Geometry: final body of the model. Coordinates: model frame, mm. Give positions to 0.01 mm unless a question says otherwise; leave off trailing zeros. Loops run counter-clockwise (first coordinate to the right, second up) from the corner with the lowest first, then second, coordinate; pieces in that order, holes last. Notation, with made-up numbers: M 37,1.25 L 74,1.25 A30 ccw 74,30.25 Z; hole C -21.75,56 d2. An arc over 180 degrees is marked long. Put each result on its own line as item: value.
```python
from build123d import *

# Parameters (mm, degrees)
DELKA_DEPTH       = 250
D_RA1_D           = 3.5
D_RA1_CBORE_D     = 6
D_RA1_CBORE_DEPTH = 4.5
LINPOLE1_COUNT    = 10
LINPOLE1_PITCH    = 25


with BuildPart() as part:
    # Skica1 → Delka (new body)
    with BuildSketch(Plane(origin=(0, 0, 0), x_dir=(1, 0, 0), z_dir=(0, 1, 0))):
        with BuildLine():
            Line((-5.5, -8), (5.5, -8))
            Line((5.5, -8), (6, -7.5))
            Line((6, -7.5), (6, -6.661895004))
            ThreePointArc((6, -6.661895004), (5.52983318, -6.420240767), (5.209128789, -6))
            Line((5.209128789, -6), (4, -5.95))
            Line((4, -5.95), (4, -5.05))
            Line((4, -5.05), (5.209128789, -5))
            ThreePointArc((5.209128789, -5), (5.52983318, -4.579759233), (6, -4.338104996))
            Line((6, -4.338104996), (6, -0.5))
            Line((6, -0.5), (5.5, 0))
            Line((5.5, 0), (-1.6, 0))
            ThreePointArc((-1.6, 0), (-2, -0.2), (-2.4, 0))
            Line((-2.4, 0), (-5.5, 0))
            Line((-5.5, 0), (-6, -0.5))
            Line((-6, -0.5), (-6, -4.338104996))
            ThreePointArc((-6, -4.338104996), (-5.52983318, -4.579759233), (-5.209128789, -5))
            Line((-5.209128789, -5), (-4, -5.05))
            Line((-4, -5.05), (-4, -5.95))
            Line((-4, -5.95), (-5.209128789, -6))
            ThreePointArc((-5.209128789, -6), (-5.52983318, -6.420240767), (-6, -6.661895004))
            Line((-6, -6.661895004), (-6, -7.5))
            Line((-6, -7.5), (-5.5, -8))
        make_face()
    extrude(amount=DELKA_DEPTH)

    # Díra1 (through all)
    with Locations(Plane.XY.offset(8)):
        with Locations((0, 12.5)):
            d_ra1 = CounterBoreHole(D_RA1_D / 2, D_RA1_CBORE_D / 2, D_RA1_CBORE_DEPTH)

    # Zkosení1: read off the stored shape, not the designer's step
    # Zkosení1 outline → Zkosení1 (revolve, cut)
    with BuildSketch(Plane.XZ.offset(-12.5)):
        Polygon((2.050001495, -1.495e-06), (1.75, 0.3), (1.75, -1.495e-06), align=None)
        Polygon((3, 8), (3, 7.7), (3.3, 8), align=None)
    zkosen_1 = revolve(axis=Axis((0, 12.5, 0), (0, 0, 1)), mode=Mode.SUBTRACT)

    # LinPole1: Díra1, Zkosení1 ×10
    with Locations(*[(0, i * LINPOLE1_PITCH, 0) for i in range(1, LINPOLE1_COUNT)]):
        add(d_ra1, mode=Mode.SUBTRACT)
        add(zkosen_1, mode=Mode.SUBTRACT)


solid = part.part
```
Item 1: Mould query, pull axis X, two halves, no side actions, for faces 1 (the flat face through (6, 123, 2)), 2 (the flat face through (0, 250, 4)), 3 (the cylindrical face through (-0.391, 215.474, 5.629)), 4 (the cylindrical face through (-0.65, 84.57, 5.63)). Classes: pulls with the +X half, pulls with the -X half, needs draft (parallel to the pull), parting line crosses it, or undercut.
Output values:
face 1: pulls with the +X half
face 2: needs draft
face 3: undercut
face 4: undercut
Item 2: Section A-A on y = 44. Output: boundary loops of the cut face in (x, z).
Output values:
outline: M -6,0.5 L -5.5,0 L -2.4,0 A0.5 cw -1.6,0 L 5.5,0 L 6,0.5 L 6,4.34 A1.2 cw 5.21,5 L 4,5.05 L 4,5.95 L 5.21,6 A1.2 cw 6,6.66 L 6,7.5 L 5.5,8 L -5.5,8 L -6,7.5 L -6,6.66 A1.2 cw -5.21,6 L -4,5.95 L -4,5.05 L -5.21,5 A1.2 cw -6,4.34 Z
Item 3: Line query: probe 1 along X at (y, z) = (112.5, 1.9); probe 2 along X at (y, z) = (62, 7); probe 3 along Z at (x, y) = (-4.5, 130). Output: solid intervals per line, ascending. Write a range as [from, to].
Output values:
probe 1: [-6, -1.75], [1.75, 6]
probe 2: [-6, -2.96], [2.96, 6]
probe 3: [0, 5.03], [5.97, 8]
Item 4: Pin query (flat end, axial travel): pin 1 Ø6 at (x, y) = (-3.5, 64) entering from -Z; pin 2 Ø3 at (x, y) = (-0.5, 87) entering from +Z; pin 3 Ø3 at (x, y) = (0, 162.5) entering from -Z. Return the tip coordinate at first contact, or that it passes through.
Output values:
pin 1: z = 0
pin 2: z = 3.5
pin 3: through
